```python
from build123d import *

# Parameters (mm, degrees)
CYLINDER001_R     = 14
CYLINDER001_DEPTH = 110
CYLINDER_R        = 28
CYLINDER_DEPTH    = 104
SKETCH_R          = 28.5
EXTRUDE_DEPTH     = 105


with BuildPart() as cylinder001:
    # Cylinder001 → Cylinder001 (new body)
    with BuildSketch(Plane.XY):
        Circle(CYLINDER001_R)
    extrude(amount=CYLINDER001_DEPTH)


with BuildPart() as cylinder:
    # Cylinder → Cylinder (new body)
    with BuildSketch(Plane.XY):
        Circle(CYLINDER_R)
    extrude(amount=CYLINDER_DEPTH)


with BuildPart() as cut001:
    # Sketch → Extrude (new body)
    with BuildSketch(Plane.XY):
        Circle(SKETCH_R)
    extrude(amount=EXTRUDE_DEPTH)

    # Cut: cut Cylinder
    add(cylinder.part, mode=Mode.SUBTRACT)

    # Cut001: cut Cylinder001
    add(cylinder001.part, mode=Mode.SUBTRACT)


solid = cut001.part
```
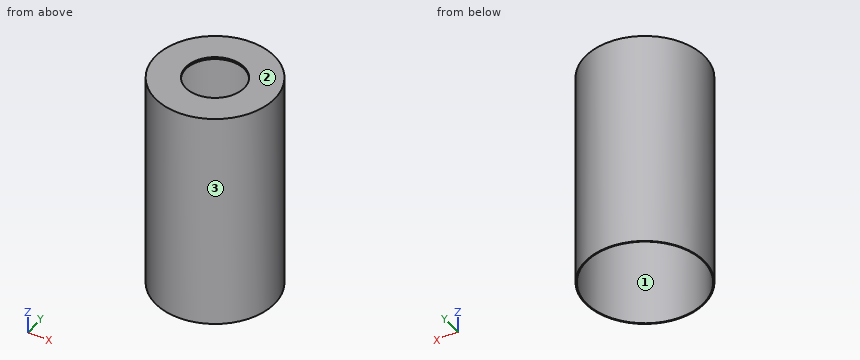
Check sheet for the modelled part. Datum: model origin and axes. Units: mm. Face numbers are marked on the shaded views. Give positions to 0.01 mm unless a question says otherwise; leave off trailing zeros. Order: outer loops, then holes, each group sorted by start corner. A loop starts at its lowest first (then second) coordinate and runs counter-clockwise, first axis right, second up. Notation, with made-up numbers: M 43.5,87 L 49.5,87 A18 ccw 49.5,97 Z; hole C 27,-27 d2. An arc over 180 degrees is marked long. Answer in a Markdown table with one row per item. Add a question column.
Q1. Gauge pin test, flat ends, axial feed: pin 1 Ø4 at (x, z) = (20, 31) entering from -Y; pin 2 Ø6 at (y, z) = (16, 17) entering from -X; pin 3 Ø2 at (x, y) = (-13, -12) entering from -Z; pin 4 Ø17 at (x, y) = (0, 0) entering from +Z. Record the tip position at first contact, or that the pin passes through.
Q2. Sectioned sample at A-A, the plane y = 0. Record the boundary of the cut face in (x, z).
Q3. Thickness scan on L1, parallel to Y at x = 0, z = 83; L2, parallel to Z at x = 14.5, y = 16; L3, parallel to Y at x = 22, z = 26.5. Record the ranges inside material, lowest first.
Q4. Sectioned sample at C-C, the plane z = 42. Record the boundary of the cut face in (x, y), and give its area (4 significant figures).
Q5. Sectioned sample at D-D, the plane y = -23. Record the boundary of the cut face in (x, z), and give its area (3 significant figures).
Q6. Release check for a two-part mould opening along Y. For the marked faces 1, 2 and 3 record: released by +Y, released by -Y, zero draft, split by the parting line, or undercut.
Verdict:
| question | item | result |
|---|---|---|
| 1 | pin 1 | y = -22.1 |
| 1 | pin 2 | x = -25.36 |
| 1 | pin 3 | z = 104 |
| 1 | pin 4 | through |
| 2 | outline | M -28.5,0 L -28,0 L -28,104 L -14,104 L -14,105 L -28.5,105 Z; M 14,104 L 28,104 L 28,0 L 28.5,0 L 28.5,105 L 14,105 Z |
| 3 | L1 | -28.5 to -28, 28 to 28.5 |
| 3 | L2 | 104 to 105 |
| 3 | L3 | -18.12 to -17.32, 17.32 to 18.12 |
| 4 | outline | C 0,0 d57; hole C 0,0 d56 |
| 4 | area | 88.75 mm² |
| 5 | outline | M -16.83,0 L -15.97,0 L -15.97,104 L 15.97,104 L 15.97,0 L 16.83,0 L 16.83,105 L -16.83,105 Z |
| 5 | area | 213 mm² |
| 6 | face 1 | undercut |
| 6 | face 2 | zero draft |
| 6 | face 3 | split by the parting line |
